from build123d import *

# Parameters (mm, degrees)
F1_DEPTH = 0.508


with BuildPart() as f1:
    # F0 (on Top) → F1 (new body)
    with BuildSketch(Plane.XY):
        with BuildLine():
            Line((-15.24, 4.7625), (0, 0))
            Line((0, 0), (25.7175, 0))
            ThreePointArc((25.7175, 0), (33.655, 7.9375), (41.5925, 0))
            Line((41.5925, 0), (67.31, 0))
            Line((67.31, 0), (68.58, 0))
            Line((68.58, 0), (73.858835, -24.13))
            Line((73.858835, -24.13), (105.211165, -24.13))
            Line((105.211165, -24.13), (110.49, 0))
            Line((110.49, 0), (111.76, 0))
            Line((111.76, 0), (111.76, -44.45))
            ThreePointArc((111.76, -44.45), (113.559583, -52.810417), (118.639583, -59.69))
            Line((118.639583, -59.69), (172.190417, -59.69))
            ThreePointArc((172.190417, -59.69), (177.270417, -52.810417), (179.07, -44.45))
            Line((179.07, -44.45), (179.07, 0))
            Line((179.07, 0), (180.34, 0))
            Line((180.34, 0), (185.618835, -24.13))
            Line((185.618835, -24.13), (216.971165, -24.13))
            Line((216.971165, -24.13), (222.25, 0))
            Line((222.25, 0), (223.52, 0))
            Line((223.52, 0), (223.52, 93.98))
            Line((223.52, 93.98), (222.25, 93.98))
            Line((222.25, 93.98), (216.971165, 118.11))
            Line((216.971165, 118.11), (185.618835, 118.11))
            Line((185.618835, 118.11), (180.34, 93.98))
            Line((180.34, 93.98), (179.07, 93.98))
            Line((179.07, 93.98), (111.76, 93.98))
            Line((111.76, 93.98), (110.49, 93.98))
            Line((110.49, 93.98), (105.211165, 118.11))
            Line((105.211165, 118.11), (73.858835, 118.11))
            Line((73.858835, 118.11), (68.58, 93.98))
            Line((68.58, 93.98), (67.31, 93.98))
            Line((67.31, 93.98), (67.31, 138.43))
            ThreePointArc((67.31, 138.43), (65.510417, 146.790417), (60.430417, 153.67))
            Line((60.430417, 153.67), (33.655, 153.67))
            Line((33.655, 153.67), (6.879583, 153.67))
            ThreePointArc((6.879583, 153.67), (1.799583, 146.790417), (0, 138.43))
            Line((0, 138.43), (0, 93.98))
            Line((0, 93.98), (-15.24, 89.2175))
            Line((-15.24, 89.2175), (-15.24, 46.99))
            Line((-15.24, 46.99), (-15.24, 4.7625))
        make_face()
    extrude(amount=F1_DEPTH)


solid = f1.part
CAD build for the part. Positions are in the model's coordinates, mm. A direction names the side the tool comes from. Round coordinates to 2 decimals unless told otherwise and drop trailing zeros. Write each loop counter-clockwise with the first axis right and the second up, starting at its lowest first coordinate (ties: lowest second). Pieces come first, ordered by that corner, then holes. Notation, with made-up numbers: M 87.25,-31 L 126.25,-31 A24 cw 126.25,-14 Z; hole C -19.75,34 d9. An arc over 180 degrees is marked long. Use a Markdown table: item, result. Add a question column.
1. Pull direction X, two halves, no side cores. Call faces 4 (the face through (65.56, 146.68, 0.25)), 5 (the face through (182.942, -11.896, 0.25)), 6 (the face through (113.51, -52.7, 0.25)): released by +X, released by -X, zero draft, split by the parting line, or undercut.
2. Slice it at A-A on y = 107. Give the cut face in (x, z), then the cut area to 3 significant figures.
3. Slice it at B-B on y = 135.5. Give the cut face in (x, z).
4. Slice it at C-C on x = 15. Give the cut face in (y, z), then the cut area to 3 significant figures.
5. 3-axis set-ups, long thin cutter, end or side, ignore diameter. For faces 1 (the face through (107.814, -12.234, 0.25)), 2 (the face through (177.22, -52.92, 0.25)), 3 (the face through (107.888, 105.876, 0.25)): which of +Z, -Z, +X, -X, +Y, -Y reach the whole face in a straight line?
6. Drill centre lines: probe 1 along X at (y, z) = (-9, 0.1); probe 2 along X at (y, z) = (-24.5, 0.3); probe 3 along X at (y, z) = (108, 0.2). Where is each one in solid material? Low to high.
Reply:
| question | item | result |
|---|---|---|
| 1 | face 4 | released by +X |
| 1 | face 5 | undercut |
| 1 | face 6 | released by -X |
| 2 | outline | M 0,0 L 67.31,0 L 67.31,0.51 L 0,0.51 Z; M 71.43,0 L 107.64,0 L 107.64,0.51 L 71.43,0.51 Z; M 183.19,0 L 219.4,0 L 219.4,0.51 L 183.19,0.51 Z |
| 2 | area | 71.0 mm^2 |
| 3 | outline | M 0,0 L 67.31,0 L 67.31,0.51 L 0,0.51 Z |
| 4 | outline | M 0,0 L 153.67,0 L 153.67,0.51 L 0,0.51 Z |
| 4 | area | 78.1 mm^2 |
| 5 | face 1 | +Z, -Z, -Y |
| 5 | face 2 | +Z, -Z, +X, -Y |
| 5 | face 3 | +Z, -Z, +Y |
| 6 | probe 1 | x = 70.55 to 108.52, 111.76 to 179.07, 182.31 to 220.28 |
| 6 | probe 2 | x = 111.76 to 179.07 |
| 6 | probe 3 | x = 0 to 67.31, 71.65 to 107.42, 183.41 to 219.18 |
